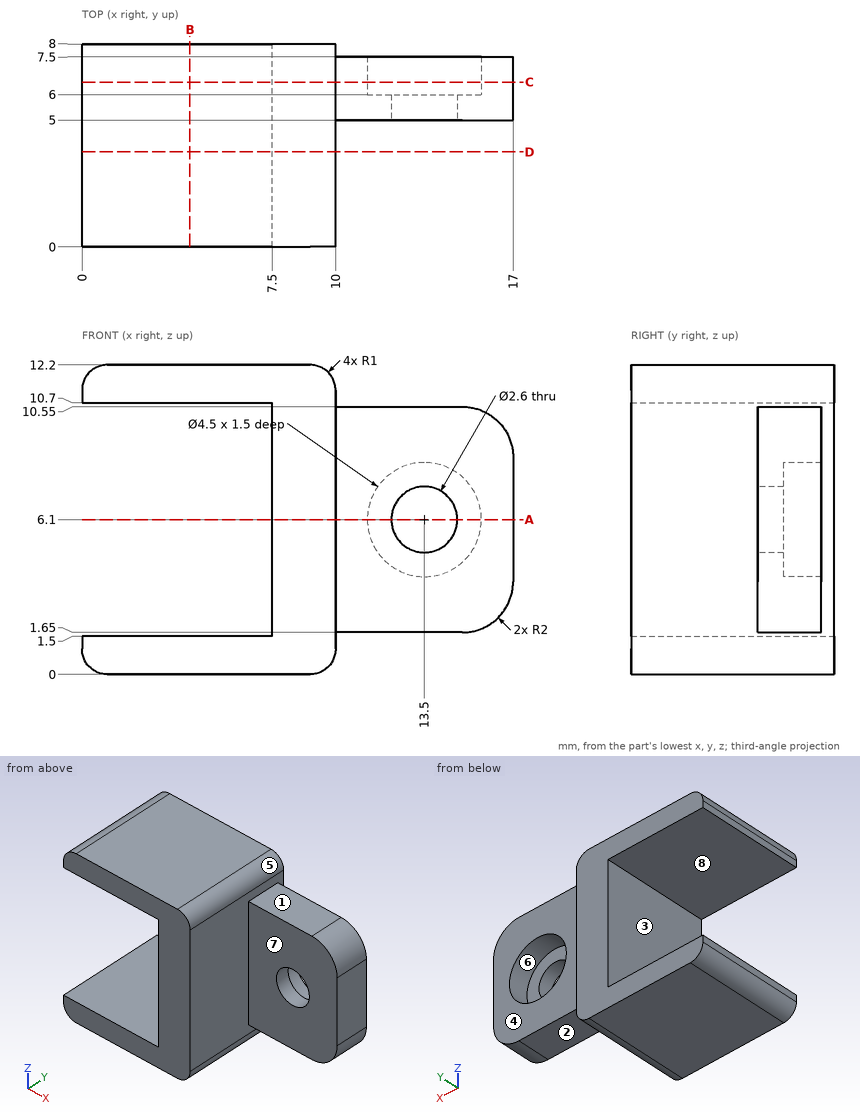
Verification items for this drawing (mm, ordinates from the low corner). A direction names the side the tool comes from. Coordinates: 2 decimals unless noted, no trailing zeros. Order: outer loops, then holes, each group sorted by start corner. A loop starts at its lowest first (then second) coordinate and runs counter-clockwise, first axis right, second up. Notation, with made-up numbers: M 63.5,-28 L 92.5,-28 A26 ccw 92.5,-8 Z; hole C 82,69 d11. An arc over 180 degrees is marked long. Answer as a JSON object with one key per item and string values.
Q1. Scan lines: line 1 (X direction, y = 7.15, z = 6.1); line 2 (Z direction, x = 13.5, y = 6.9); line 3 (X direction, y = 5.2, z = 6.1). Record each from-to range of solid material in increasing order.
Results are:
{"line 1": "x = 7.5 to 11.25, 15.75 to 17", "line 2": "z = 1.65 to 3.85, 8.35 to 10.55", "line 3": "x = 7.5 to 12.2, 14.8 to 17"}
Q2. Cross-section at A-A on z = 6.1. Record the cut outline in (x, y).
Results are:
{"outline": "M 7.5,0 L 10,0 L 10,5 L 12.2,5 L 12.2,6 L 11.25,6 L 11.25,7.5 L 10,7.5 L 10,8 L 7.5,8 Z; M 14.8,5 L 17,5 L 17,7.5 L 15.75,7.5 L 15.75,6 L 14.8,6 Z"}
Q3. Release check for a two-part mould opening along Z. For the marked faces 5, 6, 7 and 8 record: released by +Z, released by -Z, zero draft, split by the parting line, or undercut.
Results are:
{"face 5": "released by +Z", "face 6": "undercut", "face 7": "zero draft", "face 8": "undercut"}
Q4. Cross-section at B-B on x = 4.25. Record the cut outline in (y, z).
Results are:
{"outline": "M 0,0 L 8,0 L 8,1.5 L 0,1.5 Z; M 0,10.7 L 8,10.7 L 8,12.2 L 0,12.2 Z"}
Q5. Cross-section at C-C on y = 6.5. Record the cut outline in (x, z), and give its area (3 significant figures).
Results are:
{"outline": "M 0,1 A1 ccw 1,0 L 9,0 A1 ccw 10,1 L 10,1.65 L 15,1.65 A2 ccw 17,3.65 L 17,8.55 A2 ccw 15,10.55 L 10,10.55 L 10,11.2 A1 ccw 9,12.2 L 1,12.2 A1 ccw 0,11.2 L 0,10.7 L 7.5,10.7 L 7.5,1.5 L 0,1.5 Z; hole C 13.5,6.1 d4.5", "area": "96.8 mm²"}
Q6. Cross-section at D-D on y = 3.75. Record the cut outline in (x, z), and give its area (3 significant figures).
Results are:
{"outline": "M 0,1 A1 ccw 1,0 L 9,0 A1 ccw 10,1 L 10,11.2 A1 ccw 9,12.2 L 1,12.2 A1 ccw 0,11.2 L 0,10.7 L 7.5,10.7 L 7.5,1.5 L 0,1.5 Z", "area": "52.1 mm²"}
Q7. Tool access check on the marked faces 1, 2, 3 and 4. Record the directions out of +Z, -Z, +X, -X, +Y, -Y that give a thin tool (end or side, any length) a straight path to the whole face; none if there is none.
Results are:
{"face 1": "+Z, +X, +Y, -Y", "face 2": "-Z, +X, +Y, -Y", "face 3": "-X, +Y, -Y", "face 4": "+Z, -Z, +X, +Y"}
Q8. Depth check by flat-ended pin: pin 1 Ø3 at (x, y) = (12, 7) entering from -Z; pin 2 Ø6 at (x, z) = (14, 7) entering from -Y; pin 3 Ø3.5 at (x, z) = (13.5, 6.1) entering from +Y; pin 4 Ø4 at (x, y) = (6, 4.5) entering from -Z. Enter the tip coordinate at first touch or a pass-through.
Results are:
{"pin 1": "stops at z = 1.65", "pin 2": "stops at y = 5", "pin 3": "stops at y = 6", "pin 4": "stops at z = 0"}
